Input: part model. Units: mm. Frame: model coordinates. Face numbers are marked on the shaded views. A direction names the side the tool comes from. Round coordinates to 2 decimals unless told otherwise and drop trailing zeros. Order: outer loops, then holes, each group sorted by start corner. A loop starts at its lowest first (then second) coordinate and runs counter-clockwise, first axis right, second up. Notation, with made-up numbers: (-18.5, 3.25) -> (23.5, 3.25) arc R22 cw to (23.5, 24.25) -> close; hole circle Ø7 at (58.25, 64.25). An arc over 180 degrees is marked (long way). Answer as CSV lines item,"result". Start each with the question number.
1) Section query D-D, the plane x = 38. Output: boundary loops of the cut face in (y, z).
2) Line query: L1, parallel to Y at x = 25, z = 17.75; L2, parallel to X at y = 13.5, z = 22.75. Output: solid intervals per line, ascending.
3) Mould query, pull axis Y, two halves, no side actions, for the marked faces 3, 4 and 5. Classes: +Y half, -Y half, draft (parallel to the pull), parting line (faces both ways), or undercut.
4) Section query C-C, the plane x = 6. Output: boundary loops of the cut face in (y, z).
5) Section query B-B, the plane y = 37. Output: boundary loops of the cut face in (x, z), and give its area (4 significant figures).
6) Section query A-A, the plane z = 13. Output: boundary loops of the cut face in (x, y).
7) First-contact query: P1, Ø3, axis at x = 51.5, y = 67, coming from the -Z side; P2, Ø6, axis at y = 68.5, z = 4.5, coming from the +X side. Flat tips, straight axial feed; report the tip coordinate or a pass-through.
8) Access query for the marked faces 1 and 2. Directions: +Z, -Z, +X, -X, +Y, -Y. A direction counts if a zero-diameter tool reaches every point of the face in a straight line with its end or side. Return the directions, or none.
```python
from build123d import *

# Parameters (mm, degrees)
BOSS_EXTRUDE1_DEPTH            = 30
SHELL1_T                       = -5
F_3_0MM_DOWEL_HOLE1_AT_2_COUNT = 2
F_3_0MM_DOWEL_HOLE1_AT_2_PITCH = 30
F_3_0MM_DOWEL_HOLE1_AT_3_COUNT = 2
F_3_0MM_DOWEL_HOLE1_AT_3_PITCH = 32.695565449
F_3_0MM_DOWEL_HOLE1_AT_4_COUNT = 2
F_3_0MM_DOWEL_HOLE1_AT_4_PITCH = 13
BOSS_EXTRUDE2_DEPTH            = 3
SKETCH5_W                      = 55
SKETCH5_H                      = 170
CUT_EXTRUDE3_DEPTH             = 5


with BuildPart() as part:
    # Sketch1 → Boss-Extrude1 (new body)
    with BuildSketch(Plane.XY):
        Polygon((-60.491803279, 90), (60.491803279, 90), (90, 60.491803279), (90, -60.491803279), (60.491803279, -90), (-60.491803279, -90), (-90, -60.491803279), (-90, 60.491803279), align=None)
    extrude(amount=BOSS_EXTRUDE1_DEPTH)

    # Shell1
    shell1_openings = [part.faces().sort_by_distance(p)[0] for p in [
        (0, 0, 0),
    ]]
    offset(amount=SHELL1_T, openings=shell1_openings, kind=Kind.INTERSECTION)

    # Sketch3 → Ø3.0mm Dowel Hole1 (revolve, cut)
    with BuildSketch(Plane(origin=(-64.639299922, -85.852503357, 7), x_dir=(0.7071067811865476, -0.7071067811865475, 0), z_dir=(0, 0, 1))):
        Polygon((0, 0), (0, 30), (1.5, 29.098709071), (1.5, 0.025), (1.525, 0), align=None)
    f_3_0mm_dowel_hole1 = revolve(axis=Axis((-69.129427982, -90.342631418, 7), (0.7071067811865475, 0.7071067811865476, 0)), mode=Mode.SUBTRACT)

    # Ø3.0mm Dowel Hole1 at 2: Ø3.0mm Dowel Hole1 ×2
    with Locations(*[Vector(-0.7071067811865476, 0.7071067811865475, 0) * (i * F_3_0MM_DOWEL_HOLE1_AT_2_PITCH) for i in range(1, F_3_0MM_DOWEL_HOLE1_AT_2_COUNT)]):
        add(f_3_0mm_dowel_hole1, mode=Mode.SUBTRACT)

    # Ø3.0mm Dowel Hole1 at 3: Ø3.0mm Dowel Hole1 ×2
    with Locations(*[Vector(-0.6488098047725105, 0.6488098047725104, 0.3976074376343002) * (i * F_3_0MM_DOWEL_HOLE1_AT_3_PITCH) for i in range(1, F_3_0MM_DOWEL_HOLE1_AT_3_COUNT)]):
        add(f_3_0mm_dowel_hole1, mode=Mode.SUBTRACT)

    # Ø3.0mm Dowel Hole1 at 4: Ø3.0mm Dowel Hole1 ×2
    with Locations(*[(0, 0, i * F_3_0MM_DOWEL_HOLE1_AT_4_PITCH) for i in range(1, F_3_0MM_DOWEL_HOLE1_AT_4_COUNT)]):
        add(f_3_0mm_dowel_hole1, mode=Mode.SUBTRACT)

    # Mirror2: Ø3.0mm Dowel Hole1 across plane
    add(f_3_0mm_dowel_hole1.mirror(Plane.ZX), mode=Mode.SUBTRACT)

    # Mirror2 copy 1 sketch → Mirror2 copy 1 (revolve, cut)
    with BuildSketch(Plane(origin=(-85.852503357, 64.639299922, 7), x_dir=(0.7071067811865476, 0.7071067811865475, 0), z_dir=(0, 0, 1))):
        Polygon((0, 0), (0, -30), (1.5, -29.098709071), (1.5, -0.025), (1.525, 0), align=None)
    revolve(axis=Axis((-90.342631418, 69.129427982, 7), (-0.7071067811865475, 0.7071067811865476, 0)), mode=Mode.SUBTRACT)

    # Mirror2 copy 2 sketch → Mirror2 copy 2 (revolve, cut)
    with BuildSketch(Plane(origin=(-85.852503357, 64.639299922, 20), x_dir=(0.7071067811865476, 0.7071067811865475, 0), z_dir=(0, 0, 1))):
        Polygon((0, 0), (0, -30), (1.5, -29.098709071), (1.5, -0.025), (1.525, 0), align=None)
    revolve(axis=Axis((-90.342631418, 69.129427982, 20), (-0.7071067811865475, 0.7071067811865476, 0)), mode=Mode.SUBTRACT)

    # Mirror2 copy 3 sketch → Mirror2 copy 3 (revolve, cut)
    with BuildSketch(Plane(origin=(-64.639299922, 85.852503357, 20), x_dir=(0.7071067811865476, 0.7071067811865475, 0), z_dir=(0, 0, 1))):
        Polygon((0, 0), (0, -30), (1.5, -29.098709071), (1.5, -0.025), (1.525, 0), align=None)
    revolve(axis=Axis((-69.129427982, 90.342631418, 20), (-0.7071067811865475, 0.7071067811865476, 0)), mode=Mode.SUBTRACT)

    # Mirror3: Ø3.0mm Dowel Hole1 across plane
    add(f_3_0mm_dowel_hole1.mirror(Plane(origin=(0, 0, 0), x_dir=(0, 0, 1), z_dir=(1, 0, 0))), mode=Mode.SUBTRACT)

    # Mirror3 copy 1 sketch → Mirror3 copy 1 (revolve, cut)
    with BuildSketch(Plane(origin=(85.852503357, -64.639299922, 7), x_dir=(-0.7071067811865476, -0.7071067811865475, 0), z_dir=(0, 0, 1))):
        Polygon((0, 0), (0, -30), (1.5, -29.098709071), (1.5, -0.025), (1.525, 0), align=None)
    revolve(axis=Axis((90.342631418, -69.129427982, 7), (0.7071067811865475, -0.7071067811865476, 0)), mode=Mode.SUBTRACT)

    # Mirror3 copy 2 sketch → Mirror3 copy 2 (revolve, cut)
    with BuildSketch(Plane(origin=(85.852503357, -64.639299922, 20), x_dir=(-0.7071067811865476, -0.7071067811865475, 0), z_dir=(0, 0, 1))):
        Polygon((0, 0), (0, -30), (1.5, -29.098709071), (1.5, -0.025), (1.525, 0), align=None)
    revolve(axis=Axis((90.342631418, -69.129427982, 20), (0.7071067811865475, -0.7071067811865476, 0)), mode=Mode.SUBTRACT)

    # Mirror3 copy 3 sketch → Mirror3 copy 3 (revolve, cut)
    with BuildSketch(Plane(origin=(64.639299922, -85.852503357, 20), x_dir=(-0.7071067811865476, -0.7071067811865475, 0), z_dir=(0, 0, 1))):
        Polygon((0, 0), (0, -30), (1.5, -29.098709071), (1.5, -0.025), (1.525, 0), align=None)
    revolve(axis=Axis((69.129427982, -90.342631418, 20), (0.7071067811865475, -0.7071067811865476, 0)), mode=Mode.SUBTRACT)

    # Mirror3 copy 4 sketch → Mirror3 copy 4 (revolve, cut)
    with BuildSketch(Plane(origin=(64.639299922, 85.852503357, 7), x_dir=(-0.7071067811865476, 0.7071067811865475, 0), z_dir=(0, 0, 1))):
        Polygon((0, 0), (0, 30), (1.5, 29.098709071), (1.5, 0.025), (1.525, 0), align=None)
    revolve(axis=Axis((69.129427982, 90.342631418, 7), (-0.7071067811865475, -0.7071067811865476, 0)), mode=Mode.SUBTRACT)

    # Mirror3 copy 5 sketch → Mirror3 copy 5 (revolve, cut)
    with BuildSketch(Plane(origin=(85.852503357, 64.639299922, 7), x_dir=(-0.7071067811865476, 0.7071067811865475, 0), z_dir=(0, 0, 1))):
        Polygon((0, 0), (0, 30), (1.5, 29.098709071), (1.5, 0.025), (1.525, 0), align=None)
    revolve(axis=Axis((90.342631418, 69.129427982, 7), (-0.7071067811865475, -0.7071067811865476, 0)), mode=Mode.SUBTRACT)

    # Mirror3 copy 6 sketch → Mirror3 copy 6 (revolve, cut)
    with BuildSketch(Plane(origin=(85.852503357, 64.639299922, 20), x_dir=(-0.7071067811865476, 0.7071067811865475, 0), z_dir=(0, 0, 1))):
        Polygon((0, 0), (0, 30), (1.5, 29.098709071), (1.5, 0.025), (1.525, 0), align=None)
    revolve(axis=Axis((90.342631418, 69.129427982, 20), (-0.7071067811865475, -0.7071067811865476, 0)), mode=Mode.SUBTRACT)

    # Mirror3 copy 7 sketch → Mirror3 copy 7 (revolve, cut)
    with BuildSketch(Plane(origin=(64.639299922, 85.852503357, 20), x_dir=(-0.7071067811865476, 0.7071067811865475, 0), z_dir=(0, 0, 1))):
        Polygon((0, 0), (0, 30), (1.5, 29.098709071), (1.5, 0.025), (1.525, 0), align=None)
    revolve(axis=Axis((69.129427982, 90.342631418, 20), (-0.7071067811865475, -0.7071067811865476, 0)), mode=Mode.SUBTRACT)

    # Sketch4 → Boss-Extrude2 (add)
    with BuildSketch(Plane(origin=(0, 0, 25), x_dir=(-1, 0, 0), z_dir=(0, 0, -1))):
        Polygon((-58.420735467, 85), (58.420735467, 85), (85, 58.420735467), (85, -58.420735467), (58.420735467, -85), (-58.420735467, -85), (-85, -58.420735467), (-85, 58.420735467), align=None)
    extrude(amount=BOSS_EXTRUDE2_DEPTH)

    # Sketch5 → Cut-Extrude3 (cut)
    with BuildSketch(Plane(origin=(0, 0, 22), x_dir=(-1, 0, 0), z_dir=(0, 0, -1))):
        Rectangle(SKETCH5_W, SKETCH5_H)
    extrude(amount=-CUT_EXTRUDE3_DEPTH, mode=Mode.SUBTRACT)


solid = part.part
```
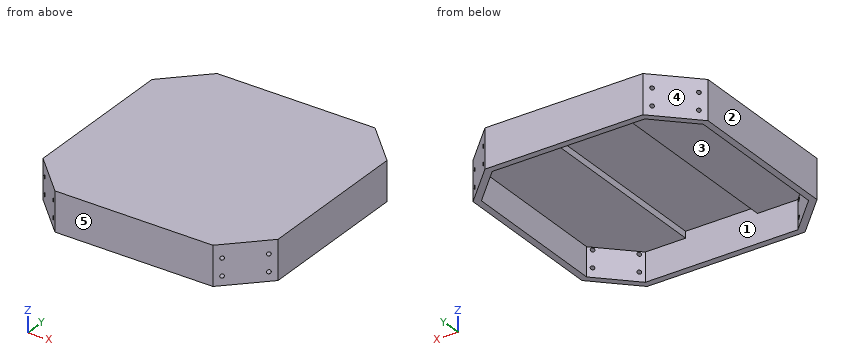
Findings:
1,outline,"(-90, 0) -> (-85, 0) -> (-85, 22) -> (85, 22) -> (85, 0) -> (90, 0) -> (90, 30) -> (-90, 30) -> close"
2,L1,"y = -90 to -85, 85 to 90"
2,L2,"x = -90 to -27.5, 27.5 to 90"
3,face 3,"undercut"
3,face 4,"+Y half"
3,face 5,"-Y half"
4,outline,"(-90, 0) -> (-85, 0) -> (-85, 27) -> (85, 27) -> (85, 0) -> (90, 0) -> (90, 30) -> (-90, 30) -> close"
5,outline,"(-90, 0) -> (-85, 0) -> (-85, 22) -> (-27.5, 22) -> (-27.5, 27) -> (27.5, 27) -> (27.5, 22) -> (85, 22) -> (85, 0) -> (90, 0) -> (90, 30) -> (-90, 30) -> close"
5,area,"1,385 mm^2"
6,outline,"(-90, -60.49) -> (-60.49, -90) -> (60.49, -90) -> (90, -60.49) -> (90, 60.49) -> (60.49, 90) -> (-60.49, 90) -> (-90, 60.49) -> close; hole (-85, -58.42) -> (-58.42, -85) -> (58.42, -85) -> (85, -58.42) -> (85, 58.42) -> (58.42, 85) -> (-58.42, 85) -> (-85, 58.42) -> close"
7,P1,"stops at z = 22"
7,P2,"stops at x = 84.99"
8,face 1,"-Z"
8,face 2,"+Z, -Z, -X, +Y, -Y"
